from build123d import *

# Parameters (mm, degrees)
F1_DEPTH = 3
F2_R     = 8.15
F3_DEPTH = 25


with BuildPart() as f1:
    # F0 (on Top) → F1 (new body)
    with BuildSketch(Plane.XY):
        with BuildLine():
            Line((0, 200), (0, 0))
            Line((0, 0), (181.761854, 0))
            Line((181.761854, 0), (163.252892, 104.96954))
            ThreePointArc((163.252892, 104.96954), (123.920575, 173.095111), (50, 200))
            Line((50, 200), (0, 200))
        make_face()
    extrude(amount=F1_DEPTH)

    # F2 (on face) → F3 (cut)
    with BuildSketch(Plane.XY.offset(3)):
        with Locations((70, 70)):
            Circle(F2_R)
    extrude(amount=-F3_DEPTH, mode=Mode.SUBTRACT)


solid = f1.part
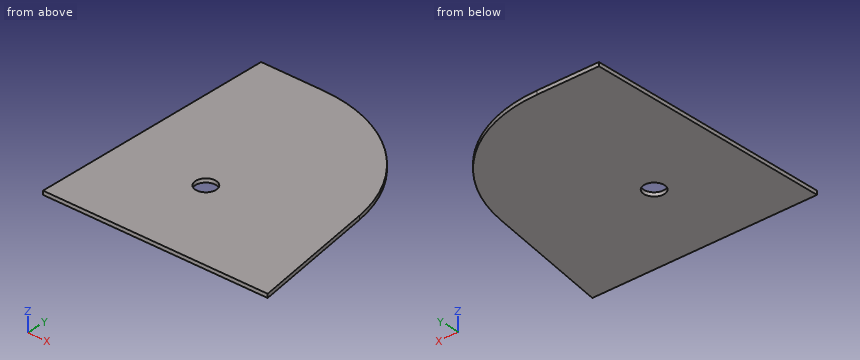
Geometry: final body of the model. Coordinates: model frame, mm. Round coordinates to 2 decimals unless told otherwise and drop trailing zeros. Loops run counter-clockwise (first coordinate to the right, second up) from the corner with the lowest first, then second, coordinate; pieces in that order, holes last. Notation, with made-up numbers: M 73,32 L 101,32 A27 cw 101,57 Z; hole C 71.5,87.25 d2. An arc over 180 degrees is marked long. Put each result on its own line as item: value. Start each with the question number.
(1) Section query B-B (x = 70). Return loops of the section in (y, z).
(2) Material intervals for line 1 along Y through (x, z) = (70, 1.1); line 2 along X through (y, z) = (66.5, 0.9); line 3 along X through (y, z) = (31.5, 2.7), sorted ascending. Write a range as [from, to].
(3) Section query D-D (y = 163). Return loops of the section in (x, z), then the cut area to 3 significant figures.
(4) Section query C-C (z = 1.9). Return loops of the section in (x, y), then the cut area to 3 significant figures.
(5) Contact query for a flat-ended pin moving along its axis: pin 1 Ø14.5 at (x, y) = (70, 70) entering from -Z. Output: stop coordinate, or through.
(6) Section query A-A (y = 70). Return loops of the section in (x, z), then the cut area to 3 significant figures.
Findings below:
1. outline: M 0,0 L 61.85,0 L 61.85,3 L 0,3 Z; M 78.15,0 L 198.25,0 L 198.25,3 L 78.15,3 Z
2. line 1: y = [0, 61.85], [78.15, 198.25]
2. line 2: x = [0, 62.64], [77.36, 170.04]
2. line 3: x = [0, 176.21]
3. outline: M 0,0 L 134.5,0 L 134.5,3 L 0,3 Z
3. area: 404 mm2
4. outline: M 0,0 L 181.76,0 L 163.25,104.97 A115 ccw 50,200 L 0,200 Z; hole C 70,70 d16.3
4. area: 30,800 mm2
5. pin 1: passes through
6. outline: M 0,0 L 61.85,0 L 61.85,3 L 0,3 Z; M 78.15,0 L 169.42,0 L 169.42,3 L 78.15,3 Z
6. area: 459 mm2
